Study the drawing (mm; zero at the part's minimum x, y, z) and answer. A direction names the side the tool comes from. Round coordinates to 2 decimals unless told otherwise and drop trailing zeros. Loops run counter-clockwise (first coordinate to the right, second up) from the corner with the lowest first, then second, coordinate; pieces in that order, holes last. Notation, with made-up numbers: (39, 84.25) - (82, 84.25) arc R38 cw to (82, 122.25) - close; hole circle Ø11 at (68.25, -34). An arc over 180 degrees is marked (long way). One line per item, written item: value.
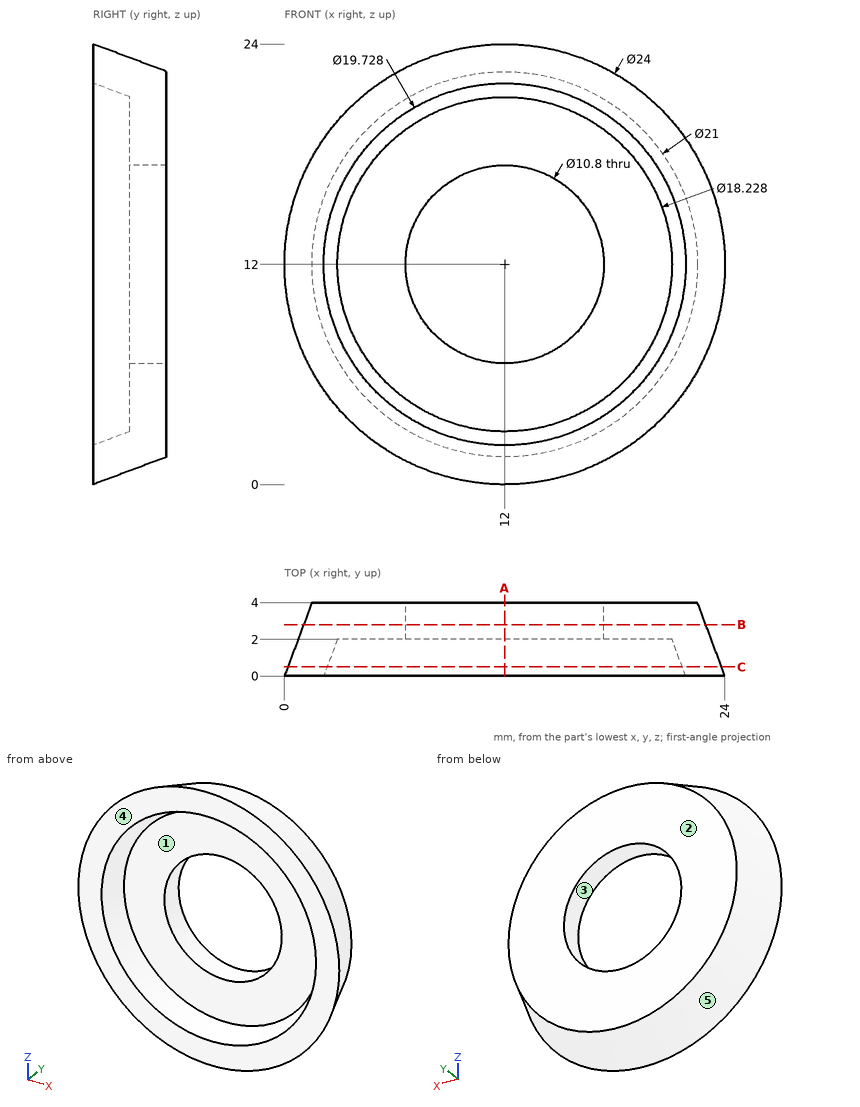
1) Consider L1, parallel to Z at x = 15, y = 2.7; L2, parallel to X at y = 0.5, z = 14.25; L3, parallel to X at y = 1.35, z = 12.5. Determine where each line is inside the solid, lowest interval first.
Final values:
L1: 1.43 to 7.51, 16.49 to 22.57
L2: 0.4 to 2.59, 21.41 to 23.6
L3: 0.52 to 2.66, 21.34 to 23.48
2) For a pull along X with two mould halves and no side action, classify the marked faces 3, 4 and 5 as released by +X, released by -X, zero draft, split by the parting line, or undercut.
Final values:
face 3: undercut
face 4: zero draft
face 5: split by the parting line
3) A cutting plane is placed at A-A on x = 12. Give the vertices of the cut face in (y, z).
Final values:
outline: (0, 0) - (4, 1.5) - (4, 6.6) - (2, 6.6) - (2, 2.89) - (0, 2.14) - close; (0, 21.86) - (2, 21.11) - (2, 17.4) - (4, 17.4) - (4, 22.5) - (0, 24) - close
4) A cutting plane is placed at C-C on y = 0.5. Give the vertices of the cut face in (x, z) (1 decimal).
Final values:
outline: circle Ø23.6 at (12, 12); hole circle Ø19.4 at (12, 12)
5) A cutting plane is placed at B-B on y = 2.8. Give the vertices of the cut face in (x, z).
Final values:
outline: circle Ø21.9 at (12, 12); hole circle Ø10.8 at (12, 12)
6) For the marked faces 1 and 2, determine the directions among +Z, -Z, +X, -X, +Y, -Y from which every point of the face is accessible in a straight line to the end or side of a thin tool.
Final values:
face 1: -Y
face 2: +Z, -Z, +X, -X, +Y
